The model under review builds one solid part; all positions refer to its coordinate system, in mm. Face numbers are marked on the shaded views. A direction names the side the tool comes from. Round coordinates to 2 decimals unless told otherwise and drop trailing zeros. Write each loop counter-clockwise with the first axis right and the second up, starting at its lowest first coordinate (ties: lowest second). Pieces come first, ordered by that corner, then holes. Notation, with made-up numbers: M 80.5,52 L 130.5,52 A24 ccw 130.5,85 Z; hole C -11,-18 d2. An arc over 180 degrees is marked long. One line per item, written item: value. Start each with the question number.
1) Take a section at A-A, the plane y = -1. Write out the cut boundary in (x, z) (1 decimal).
2) Mouldability with a two-part tool opening along X and no side actions: class the marked faces 1, 2 and 3 as +X half, -X half, draft (parallel to the pull), parting line (faces both ways), or undercut.
3) Take a section at C-C, the plane y = 5.5. State how many separate pieces and enclosed holes the cut face has, and give its area (3 significant figures).
4) For P1, Ø1.8, axis at x = -22.5, z = 0, coming from the -Y side; P2, Ø2.5, axis at x = -48.5, z = 0, coming from the +Y side; P3, Ø3, axis at x = 8.5, y = 1, coming from the +Z side; P4, Ø10, axis at x = -36.5, y = 6, coming from the -Z side, all flat-tipped, find the tip position at first contact; note any pin that passes through.
5) Take a section at B-B, the plane x = 0. Write out the cut boundary in (y, z), and give its area (3 significant figures).
6) Wall thickness on probe 1 along Z at (x, y) = (-48.5, 0); probe 2 along X at (y, z) = (-14, -0.75); probe 3 along Z at (x, y) = (21, 4.5): over which ranges is each line inside the solid? List them lowest first.
7) Tool access review of the marked faces 4, 5, 6 and 7: name each direction out of +Z, -Z, +X, -X, +Y, -Y from which nothing blocks a thin tool from reaching the whole face with its end or side.
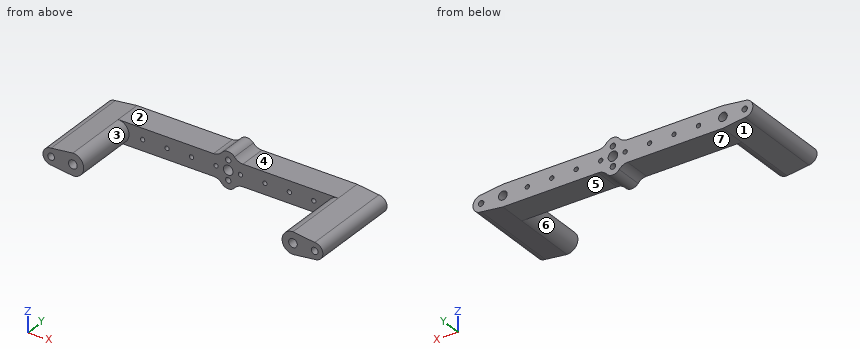
from build123d import *

# Parameters (mm, degrees)
SKETCH1_R                 = 1.5875
SKETCH1_R_2               = 1
BOSS_EXTRUDE1_DEPTH       = 24
BOSS_EXTRUDE1_2_DEPTH     = 24
BOSS_EXTRUDE2_START       = 10
SKETCH2_R                 = 0.79375
SKETCH2_R_2               = 1.5875
SKETCH2_R_3               = 1
SKETCH2_R_4               = 1.75
BOSS_EXTRUDE2_DEPTH       = 10
M3X0_5_TAPPED_HOLE1_D     = 2.5
M3X0_5_TAPPED_HOLE1_DEPTH = 18.5
M3X0_5_TAPPED_HOLE1_TIP   = 0.751075774


with BuildPart() as part:
    # Sketch1 → Boss-Extrude1 (new body)
    with BuildSketch(Plane(origin=(0, 0, 0), x_dir=(1, 0, 0), z_dir=(0, 1, 0))):
        with BuildLine():
            Line((-40.5, 4), (-48.5, 3))
            ThreePointArc((-48.5, 3), (-51.5, 0), (-48.5, -3))
            Line((-48.5, -3), (-40.5, -4))
            ThreePointArc((-40.5, -4), (-36.5, 0), (-40.5, 4))
        make_face()
        with Locations(Location((-40.5, 0, 0), (0, 0, 270))):
            Circle(SKETCH1_R, mode=Mode.SUBTRACT)
        with Locations(Location((-48.5, 0, 0), (0, 0, 270))):
            Circle(SKETCH1_R_2, mode=Mode.SUBTRACT)
    extrude(amount=-BOSS_EXTRUDE1_DEPTH)



with BuildPart() as body_2:
    # Sketch1 → Boss-Extrude1 2 (new body)
    with BuildSketch(Plane(origin=(0, 0, 0), x_dir=(1, 0, 0), z_dir=(0, 1, 0))):
        with BuildLine():
            Line((48.5, -3), (40.5, -4))
            ThreePointArc((40.5, -4), (36.5, 0), (40.5, 4))
            Line((40.5, 4), (48.5, 3))
            ThreePointArc((48.5, 3), (51.5, 0), (48.5, -3))
        make_face()
        with Locations(Location((40.5, 0, 0), (0, 0, 90))):
            Circle(SKETCH1_R, mode=Mode.SUBTRACT)
        with Locations(Location((48.5, 0, 0), (0, 0, 90))):
            Circle(SKETCH1_R_2, mode=Mode.SUBTRACT)
    extrude(amount=-BOSS_EXTRUDE1_2_DEPTH)


with BuildPart() as part_1:
    add(part.part)

    add(body_2.part)  # Boss-Extrude2 merges body 2
    # Sketch2 → Boss-Extrude2 (add)
    with BuildSketch(Plane(origin=(0, 0, 0), x_dir=(1, 0, 0), z_dir=(0, 1, 0)).offset(BOSS_EXTRUDE2_START)):
        with BuildLine():
            Line((-40.5, 4), (-48.5, 3))
            ThreePointArc((-48.5, 3), (-51.5, 0), (-48.5, -3))
            Line((-48.5, -3), (-40.5, -4))
            Line((-40.5, -4), (-5.427594702, -4))
            ThreePointArc((-5.427594702, -4), (-3.710635508, -4.387237743), (-2.326112015, -5.473974438))
            ThreePointArc((-2.326112015, -5.473974438), (0, -6.579455266), (2.326112015, -5.473974438))
            ThreePointArc((2.326112015, -5.473974438), (3.710635508, -4.387237743), (5.427594702, -4))
            Line((5.427594702, -4), (40.5, -4))
            Line((40.5, -4), (48.5, -3))
            ThreePointArc((48.5, -3), (51.5, 0), (48.5, 3))
            Line((48.5, 3), (40.5, 4))
            Line((40.5, 4), (5.427594702, 4))
            ThreePointArc((5.427594702, 4), (3.710635508, 4.387237743), (2.326112015, 5.473974438))
            ThreePointArc((2.326112015, 5.473974438), (0, 6.579455266), (-2.326112015, 5.473974438))
            ThreePointArc((-2.326112015, 5.473974438), (-3.710635508, 4.387237743), (-5.427594702, 4))
            Line((-5.427594702, 4), (-40.5, 4))
        make_face()
        with Locations(Location((-31.5, 0, 0), (0, 0, 270))):
            Circle(SKETCH2_R, mode=Mode.SUBTRACT)
        with Locations(Location((-22.5, 0, 0), (0, 0, 270))):
            Circle(SKETCH2_R, mode=Mode.SUBTRACT)
        with Locations(Location((-40.5, 0, 0), (0, 0, 270))):
            Circle(SKETCH2_R_2, mode=Mode.SUBTRACT)
        with Locations(Location((40.5, 0, 0), (0, 0, 90))):
            Circle(SKETCH2_R_2, mode=Mode.SUBTRACT)
        with Locations(Location((-13.5, 0, 0), (0, 0, 270))):
            Circle(SKETCH2_R, mode=Mode.SUBTRACT)
        with Locations(Location((-4.5, 0, 0), (0, 0, 270))):
            Circle(SKETCH2_R, mode=Mode.SUBTRACT)
        with Locations(Location((4.5, 0, 0), (0, 0, 270))):
            Circle(SKETCH2_R, mode=Mode.SUBTRACT)
        with Locations(Location((13.5, 0, 0), (0, 0, 270))):
            Circle(SKETCH2_R, mode=Mode.SUBTRACT)
        with Locations(Location((22.5, 0, 0), (0, 0, 270))):
            Circle(SKETCH2_R, mode=Mode.SUBTRACT)
        with Locations(Location((31.5, 0, 0), (0, 0, 270))):
            Circle(SKETCH2_R, mode=Mode.SUBTRACT)
        with Locations(Location((48.5, 0, 0), (0, 0, 90))):
            Circle(SKETCH2_R_3, mode=Mode.SUBTRACT)
        with Locations(Location((-48.5, 0, 0), (0, 0, 270))):
            Circle(SKETCH2_R_3, mode=Mode.SUBTRACT)
        with Locations(Location((0, 0, 0), (0, 0, 270))):
            Circle(SKETCH2_R_4, mode=Mode.SUBTRACT)
        with Locations(Location((0, -3.579455266, 0), (0, 0, 270))):
            Circle(SKETCH2_R_3, mode=Mode.SUBTRACT)
        with Locations(Location((0, 3.579455266, 0), (0, 0, 270))):
            Circle(SKETCH2_R_3, mode=Mode.SUBTRACT)
    extrude(amount=-BOSS_EXTRUDE2_DEPTH)

    # M3x0.5 Tapped Hole1
    with Locations(Plane(origin=(-48.5, -24, 0), x_dir=(0, 0, -1), z_dir=(0, -1, 0))):
        with Locations((0, 0), (0, 97)):
            Hole(M3X0_5_TAPPED_HOLE1_D / 2, depth=M3X0_5_TAPPED_HOLE1_DEPTH)
            with Locations((0, 0, -(M3X0_5_TAPPED_HOLE1_DEPTH + M3X0_5_TAPPED_HOLE1_TIP / 2))):  # 118° drill point
                Cone(0, M3X0_5_TAPPED_HOLE1_D / 2, M3X0_5_TAPPED_HOLE1_TIP, mode=Mode.SUBTRACT)


solid = part_1.part
Checked values:
1. outline: M -48.5,-3 L -40.5,-4 A4 ccw -40.5,4 L -48.5,3 A3 ccw Z; M 40.5,-4 L 48.5,-3 A3 ccw 48.5,3 L 40.5,4 A4 ccw Z; hole C -48.5,0 d2; hole C -40.5,0 d3.2; hole C 40.5,0 d3.2; hole C 48.5,0 d2
2. face 1: -X half
2. face 2: draft
2. face 3: undercut
3. separate pieces: 1
3. enclosed holes: 15
3. area: 761 mm2
4. P1: stops at y = 0
4. P2: stops at y = 10
4. P3: stops at z = 4
4. P4: stops at z = -4
5. outline: M 0,-6.58 L 10,-6.58 L 10,-4.58 L 0,-4.58 Z; M 0,-2.58 L 10,-2.58 L 10,-1.75 L 0,-1.75 Z; M 0,1.75 L 10,1.75 L 10,2.58 L 0,2.58 Z; M 0,4.58 L 10,4.58 L 10,6.58 L 0,6.58 Z
5. area: 56.6 mm2
6. probe 1: z = -3 to -1, 1 to 3
6. probe 2: x = -51.4 to -49.5, -47.5 to -41.9, -39.1 to -36.57, 36.57 to 39.1, 41.9 to 47.5, 49.5 to 51.4
6. probe 3: z = -4 to 4
7. face 4: +Z, +X, +Y, -Y
7. face 5: -Z, +X, +Y, -Y
7. face 6: -Y
7. face 7: -Z, -X, +Y, -Y
